Could you check a few things on this drawing? It's one solid part, dimensions in mm from its lowest x, y, z. Coordinates: 2 decimals unless noted, no trailing zeros. Loops run counter-clockwise (first coordinate to the right, second up) from the corner with the lowest first, then second, coordinate; pieces in that order, holes last.
1) Imagine slicing it at B-B on x = 8.25. Please give me the cut outline in (y, z).
2) If I drill on line 1 along Y through (x, z) = (7.75, 3.5); line 2 along Z through (x, y) = (7.25, 0.5); line 3 along Y through (x, z) = (0.5, 1.5), over which ranges is the centre line in solid material (lowest first)?
3) Imagine slicing it at C-C on y = 0.4. Please give me the cut outline in (x, z).
4) Imagine slicing it at A-A on z = 1.75. Please give me the cut outline in (x, y), plus the area to 3 significant figures.
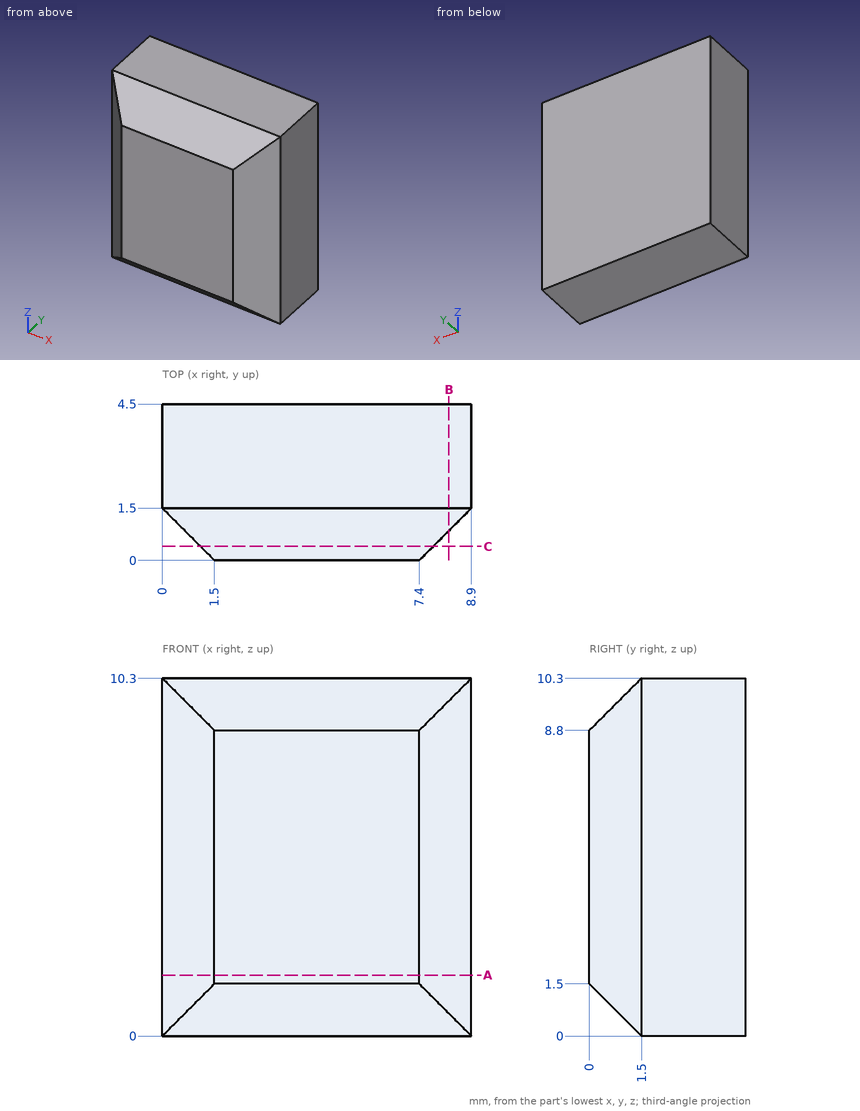
Filled in:
1. outline: (0.85, 0.65) - (1.5, 0) - (4.5, 0) - (4.5, 10.3) - (1.5, 10.3) - (0.85, 9.65) - close
2. line 1: y = 0.35 to 4.5
2. line 2: z = 1 to 9.3
2. line 3: y = 1 to 4.5
3. outline: (1.1, 1.1) - (7.8, 1.1) - (7.8, 9.2) - (1.1, 9.2) - close
4. outline: (0, 1.5) - (1.5, 0) - (7.4, 0) - (8.9, 1.5) - (8.9, 4.5) - (0, 4.5) - close
4. area: 37.8 mm2
